Verification items for the finished model (mm, model axes). A direction names the side the tool comes from. Coordinates: 2 decimals unless noted, no trailing zeros. Loops run counter-clockwise (first coordinate to the right, second up) from the corner with the lowest first, then second, coordinate; pieces in that order, holes last. Notation, with made-up numbers: (21, 54) -> (56, 54) arc R21 cw to (56, 69) -> close; hole circle Ø3 at (67.5, 36.5). An arc over 180 degrees is marked (long way). Answer as a JSON object with one key per item and string values. Group by question number.
Q1. Set-up check for faces 1 (the cylindrical face through (4, 7, 0)), 2 (the flat face through (5, -2, 0)), 3 (the flat face through (2, -2, 2)): record each of +Z, -Z, +X, -X, +Y, -Y from which the full face is reachable in a straight line by a thin tool's end or side.
Q2. Cross-section at A-A on x = 2.25. Record the boundary of the cut face in (y, z).
Q3. Gauge pin test, flat ends, axial feed: pin 1 Ø2 at (x, z) = (2.5, 7) entering from -Y; pin 2 Ø2 at (x, z) = (4, -6.5) entering from +Y; pin 3 Ø2.5 at (y, z) = (6, 0) entering from -X; pin 4 Ø1.8 at (y, z) = (3, 5.2) entering from -X. Record the tip position at first contact, or that the pin passes through.
Q4. Cross-section at D-D on y = 3. Record the boundary of the cut face in (x, z), and give its area (3 significant figures).
Q5. Scan lines: L1, parallel to Y at x = 4.1, z = 0; L2, parallel to X at y = -5.75, z = 6.75; L3, parallel to X at y = 7, z = -1.75. Record each from-to range of solid material in increasing order.
Q6. Release check for a two-part mould opening along Z. For faces 4 (the cylindrical face through (4, -5, 0)), 5 (the cylindrical face through (0.99, -8.43, 4.38)), 6 (the flat face through (0, -1, -1)), 7 (the cylindrical face through (3.5, 3.2, -10)) record: released by +Z, released by -Z, zero draft, split by the parting line, or undercut.
Q7. Cross-section at C-C on z = 0. Record the boundary of the cut face in (x, y), and give its area (3 significant figures).
Q8. Cross-section at B-B on y = 0. Record the boundary of the cut face in (x, z), and give its area (3 significant figures).
```python
from build123d import *

# Parameters (mm, degrees)
SKETCH1_R           = 10.5
BOSS_EXTRUDE1_DEPTH = 7
SKETCH2_R           = 7.5
CUT_EXTRUDE1_DEPTH  = 2
SKETCH3_R           = 1
CUT_EXTRUDE2_DEPTH  = 6
SKETCH4_R           = 9.5
SKETCH4_R_2         = 2.5
CUT_EXTRUDE3_DEPTH  = 2


with BuildPart() as part:
    # Sketch1 → Boss-Extrude1 (new body)
    with BuildSketch(Plane(origin=(0, 0, 0), x_dir=(0, 0, -1), z_dir=(1, 0, 0))):
        Circle(SKETCH1_R)
    extrude(amount=BOSS_EXTRUDE1_DEPTH)

    # Sketch2 → Cut-Extrude1 (cut)
    with BuildSketch(Plane(origin=(7, 0, 0), x_dir=(0, 0, -1), z_dir=(1, 0, 0))):
        Circle(SKETCH2_R)
    extrude(amount=-CUT_EXTRUDE1_DEPTH, mode=Mode.SUBTRACT)

    # Sketch3 → Cut-Extrude2 (cut, through all)
    with BuildSketch(Plane(origin=(5, 0, 0), x_dir=(0, 0, -1), z_dir=(1, 0, 0))):
        with Locations((0, 6)):
            Circle(SKETCH3_R)
        Circle(SKETCH3_R)
        with Locations((5.196152423, 3)):
            Circle(SKETCH3_R)
        with Locations((5.196152423, -3)):
            Circle(SKETCH3_R)
        with Locations((0, -6)):
            Circle(SKETCH3_R)
        with Locations((-5.196152423, -3)):
            Circle(SKETCH3_R)
        with Locations((-5.196152423, 3)):
            Circle(SKETCH3_R)
    extrude(amount=-CUT_EXTRUDE2_DEPTH, mode=Mode.SUBTRACT)

    # Sketch4 → Cut-Extrude3 (cut)
    with BuildSketch(Plane.ZY):
        Circle(SKETCH4_R)
        Circle(SKETCH4_R_2, mode=Mode.SUBTRACT)
    extrude(amount=-CUT_EXTRUDE3_DEPTH, mode=Mode.SUBTRACT)


solid = part.part
```
Computed values:
{
 "1": {"face 1": "+X, -X", "face 2": "+X", "face 3": "-X"},
 "2": {"outline": "circle Ø21 at (0, 0); hole circle Ø2 at (-6, 0); hole circle Ø2 at (-3, -5.2); hole circle Ø2 at (-3, 5.2); hole circle Ø2 at (0, 0); hole circle Ø2 at (3, -5.2); hole circle Ø2 at (3, 5.2); hole circle Ø2 at (6, 0)"},
 "3": {"pin 1": "stops at y = -8.62", "pin 2": "stops at y = 8.94", "pin 3": "stops at x = 2", "pin 4": "passes through"},
 "4": {"outline": "(0, -10.06) -> (7, -10.06) -> (7, -6.87) -> (5, -6.87) -> (5, -6.2) -> (2, -6.2) -> (2, -9.01) -> (0, -9.01) -> close; (0, 9.01) -> (2, 9.01) -> (2, 6.2) -> (5, 6.2) -> (5, 6.87) -> (7, 6.87) -> (7, 10.06) -> (0, 10.06) -> close; (2, -4.2) -> (5, -4.2) -> (5, 4.2) -> (2, 4.2) -> close", "area": "65.3 mm²"},
 "5": {"L1": "y = -10.5 to -7, -5 to -1, 1 to 5, 7 to 10.5", "L2": "x = 2 to 7", "L3": "x = 2 to 5"},
 "6": {"face 4": "undercut", "face 5": "undercut", "face 6": "zero draft", "face 7": "split by the parting line"},
 "7": {"outline": "(0, -10.5) -> (7, -10.5) -> (7, -7.5) -> (5, -7.5) -> (5, -7) -> (2, -7) -> (2, -9.5) -> (0, -9.5) -> close; (0, -2.5) -> (2, -2.5) -> (2, -5) -> (5, -5) -> (5, -1) -> (0, -1) -> close; (0, 1) -> (5, 1) -> (5, 5) -> (2, 5) -> (2, 2.5) -> (0, 2.5) -> close; (0, 9.5) -> (2, 9.5) -> (2, 7) -> (5, 7) -> (5, 7.5) -> (7, 7.5) -> (7, 10.5) -> (0, 10.5) -> close", "area": "67.0 mm²"},
 "8": {"outline": "(0, -10.5) -> (7, -10.5) -> (7, -7.5) -> (5, -7.5) -> (5, -1) -> (0, -1) -> (0, -2.5) -> (2, -2.5) -> (2, -9.5) -> (0, -9.5) -> close; (0, 1) -> (5, 1) -> (5, 7.5) -> (7, 7.5) -> (7, 10.5) -> (0, 10.5) -> (0, 9.5) -> (2, 9.5) -> (2, 2.5) -> (0, 2.5) -> close", "area": "79.0 mm²"}
}
